```python
from build123d import *

# Parameters (mm, degrees)
SKETCH1_R           = 1
SKETCH1_R_2         = 1.825
BOSS_EXTRUDE1_DEPTH = 3.175


with BuildPart() as part:
    # Sketch1 → Boss-Extrude1 (new body)
    with BuildSketch(Plane.XY):
        Polygon((0, 8), (0, 0), (0, -12), (28.35, -12), (28.35, 8), (23.85, 8), (23.85, 0), (4.5, 0), (4.5, 8), align=None)
        with Locations((2.75, 4)):
            Circle(SKETCH1_R, mode=Mode.SUBTRACT)
        with Locations((25.6, 4)):
            Circle(SKETCH1_R, mode=Mode.SUBTRACT)
        with Locations((6, -7)):
            Circle(SKETCH1_R_2, mode=Mode.SUBTRACT)
        with Locations((22.35, -7)):
            Circle(SKETCH1_R_2, mode=Mode.SUBTRACT)
    extrude(amount=BOSS_EXTRUDE1_DEPTH)


solid = part.part
```
Here's how the part is built. I have some questions about the finished solid (model axes, mm). A direction names the side the tool comes from. Coordinates: 2 decimals unless noted, no trailing zeros. Loops run counter-clockwise (first coordinate to the right, second up) from the corner with the lowest first, then second, coordinate; pieces in that order, holes last. Notation, with made-up numbers: (-7.75, -38) -> (19.25, -38) arc R21 ccw to (19.25, -22) -> close; hole circle Ø7 at (-24, -28). An arc over 180 degrees is marked (long way). Return JSON: item names as keys, results as strings.
1) If we section it at B-B, the plane x = 2.75: Write out the boundary of the cut face in (y, z) (3 decimals).
Results below:
{"outline": "(-12, 0) -> (3, 0) -> (3, 3.175) -> (-12, 3.175) -> close; (5, 0) -> (8, 0) -> (8, 3.175) -> (5, 3.175) -> close"}
2) If we section it at C-C, the plane y = 0.75: Write out the boundary of the cut face in (x, z) (3 decimals).
Results below:
{"outline": "(0, 0) -> (4.5, 0) -> (4.5, 3.175) -> (0, 3.175) -> close; (23.85, 0) -> (28.35, 0) -> (28.35, 3.175) -> (23.85, 3.175) -> close"}
3) If we section it at D-D, the plane z = 2.35: Write out the boundary of the cut face in (x, y) (3 decimals), then the cut area to 3 significant figures.
Results below:
{"outline": "(0, -12) -> (28.35, -12) -> (28.35, 8) -> (23.85, 8) -> (23.85, 0) -> (4.5, 0) -> (4.5, 8) -> (0, 8) -> close; hole circle Ø2 at (2.75, 4); hole circle Ø3.65 at (6, -7); hole circle Ø3.65 at (22.35, -7); hole circle Ø2 at (25.6, 4)", "area": "385 mm²"}
4) I need wall thicknesses on line 1 (Y direction, x = 6, z = 1.1) (3 decimals); line 2 (X direction, y = 0.5, z = 2.6); line 3 (X direction, y = -5.5, z = 2.15). Which ranges of each line are inside material? Lowest first, please. Write a range as from..to.
Results below:
{"line 1": "-12..-8.825, -5.175..0", "line 2": "0..4.5, 23.85..28.35", "line 3": "0..4.96, 7.04..21.31, 23.39..28.35"}
5) For faces 1 (the face through (28.35, -2, 2)), 2 (the face through (23.85, 4, 2)), which set-ups out of +Z, -Z, +X, -X, +Y, -Y let a thin tool reach every point of the face, with its end or its side?
Results below:
{"face 1": "+Z, -Z, +X, +Y, -Y", "face 2": "+Z, -Z, +Y"}
6) Thinking about a two-plate mould opening in X: for faces 3 (the face through (0, -2, 2)), 4 (the face through (24.09, -6.45, 1.57)), 5 (the face through (14, -4, 0)), which applies, +X half, -X half, draft (parallel to the pull), parting line (faces both ways), or undercut?
Results below:
{"face 3": "-X half", "face 4": "undercut", "face 5": "draft"}
7) If we section it at A-A, the plane y = -7: Write out the boundary of the cut face in (x, z) (3 decimals), then the cut area to 3 significant figures.
Results below:
{"outline": "(0, 0) -> (4.175, 0) -> (4.175, 3.175) -> (0, 3.175) -> close; (7.825, 0) -> (20.525, 0) -> (20.525, 3.175) -> (7.825, 3.175) -> close; (24.175, 0) -> (28.35, 0) -> (28.35, 3.175) -> (24.175, 3.175) -> close", "area": "66.8 mm²"}
8) Will this pin go through, and if not, where does the flat tip stop? pin 1 (1.6 mm diameter, centred on x = 12, z = 2.5, fed in from +Y).
Results below:
{"pin 1": "y = 0"}
